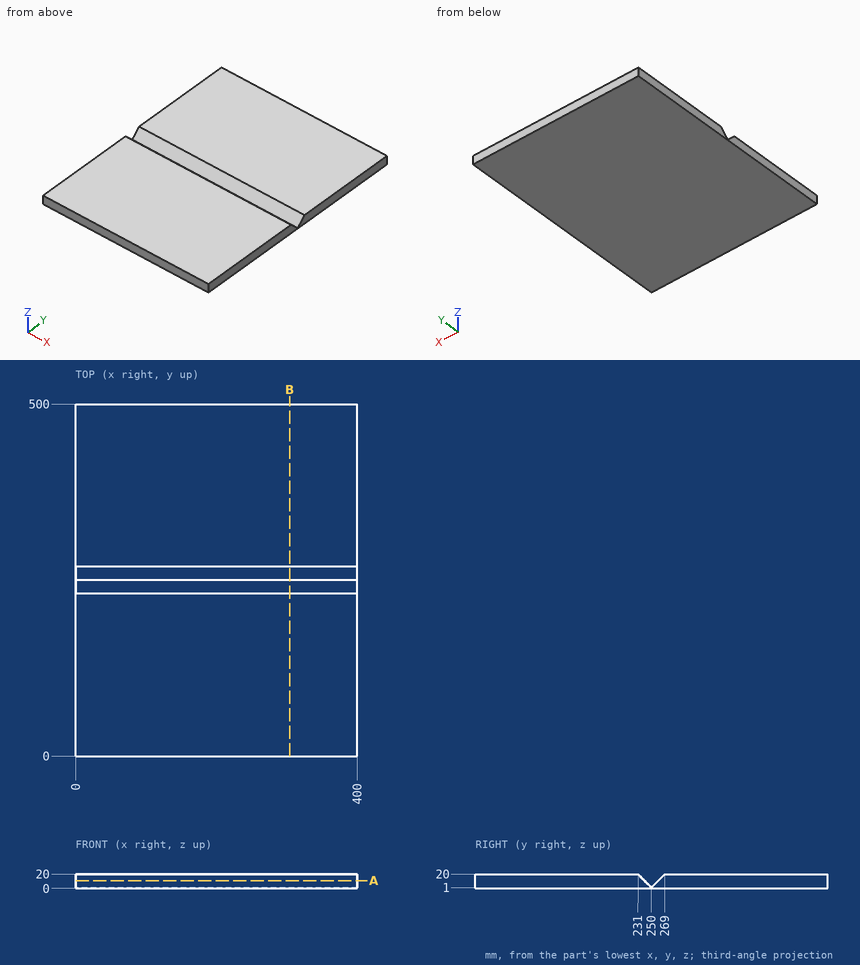
Job drawing, mm, ordinate dimensions from the low corner. One solid piece. Coordinates: 2 decimals unless noted, no trailing zeros. Order: outer loops, then holes, each group sorted by start corner. A loop starts at its lowest first (then second) coordinate and runs counter-clockwise, first axis right, second up. Notation, with made-up numbers: (47, 8) -> (94, 8) arc R35 cw to (94, 43) -> close; hole circle Ø2 at (17, 31.5). An arc over 180 degrees is marked (long way). Put each result on its own line as item: value. Start each with the question number.
(1) Pin check, flat tip, straight feed: pin 1 Ø1 at (y, z) = (257, 11) entering from +X. Stop position of the tip, or through.
(2) Probe line 1 along Y through (x, z) = (46, 11.75); line 2 along Y through (x, z) = (156.5, 9.25). List the from-to ranges inside material, lowest first. Write a range as [from, to].
(3) Band-saw the part on B-B (x = 304). Give the cut face in (y, z), then the cut area to 3 significant figures.
(4) Band-saw the part on A-A (z = 11). Give the cut face in (x, y), then the cut area to 3 significant figures.
Determined:
1. pin 1: passes through
2. line 1: y = [0, 239.25], [260.75, 500]
2. line 2: y = [0, 241.75], [258.25, 500]
3. outline: (0, 0) -> (500, 0) -> (500, 20) -> (269, 20) -> (250, 1) -> (231, 20) -> (0, 20) -> close
3. area: 9,640 mm²
4. outline: (0, 0) -> (400, 0) -> (400, 240) -> (0, 240) -> close; (0, 260) -> (400, 260) -> (400, 500) -> (0, 500) -> close
4. area: 192,000 mm²
